```python
from build123d import *

# Parameters (mm, degrees)
BOSS_EXTRUDE1_DEPTH = 2.5
BOSS_EXTRUDE3_START = 2.5
BOSS_EXTRUDE3_DEPTH = 3
BOSS_EXTRUDE2_DEPTH = 7


with BuildPart() as part:
    # Sketch1 → Boss-Extrude1 (new body)
    with BuildSketch(Plane.XY):
        with BuildLine():
            ThreePointArc((-43.2, -11.688179282), (-41.735533906, -15.223713187), (-38.2, -16.688179282))
            Line((-38.2, -16.688179282), (-5, -16.688179282))
            Line((-5, -16.688179282), (-5, 5.203986913))
            Line((-5, 5.203986913), (-35.346679904, 16.688179282))
            Line((-35.346679904, 16.688179282), (-38.2, 16.688179282))
            ThreePointArc((-38.2, 16.688179282), (-41.735533906, 15.223713187), (-43.2, 11.688179282))
            Line((-43.2, 11.688179282), (-43.2, -11.688179282))
        make_face()
        with BuildLine():
            ThreePointArc((-41.2, 11.338179282), (-37.85, 14.688179282), (-34.5, 11.338179282))
            Line((-34.5, 11.338179282), (-34.5, 1.338179282))
            ThreePointArc((-34.5, 1.338179282), (-37.85, -2.011820718), (-41.2, 1.338179282))
            Line((-41.2, 1.338179282), (-41.2, 11.338179282))
        make_face(mode=Mode.SUBTRACT)
        with BuildLine():
            Line((-41.2, 11.338179282), (-41.2, 1.338179282))
            ThreePointArc((-41.2, 1.338179282), (-37.85, -2.011820718), (-34.5, 1.338179282))
            Line((-34.5, 1.338179282), (-34.5, 11.338179282))
            ThreePointArc((-34.5, 11.338179282), (-37.85, 14.688179282), (-41.2, 11.338179282))
        make_face()
        with BuildLine():
            Line((5, 5.203986913), (5, -16.688179282))
            Line((5, -16.688179282), (38.2, -16.688179282))
            ThreePointArc((38.2, -16.688179282), (41.735533906, -15.223713187), (43.2, -11.688179282))
            Line((43.2, -11.688179282), (43.2, 11.688179282))
            ThreePointArc((43.2, 11.688179282), (41.735533906, 15.223713187), (38.2, 16.688179282))
            Line((38.2, 16.688179282), (35.346679904, 16.688179282))
            Line((35.346679904, 16.688179282), (5, 5.203986913))
        make_face()
        with BuildLine():
            ThreePointArc((34.5, 11.338179282), (37.85, 14.688179282), (41.2, 11.338179282))
            Line((41.2, 11.338179282), (41.2, 1.338179282))
            ThreePointArc((41.2, 1.338179282), (37.85, -2.011820718), (34.5, 1.338179282))
            Line((34.5, 1.338179282), (34.5, 11.338179282))
        make_face(mode=Mode.SUBTRACT)
        with BuildLine():
            Line((34.5, 11.338179282), (34.5, 1.338179282))
            ThreePointArc((34.5, 1.338179282), (37.85, -2.011820718), (41.2, 1.338179282))
            Line((41.2, 1.338179282), (41.2, 11.338179282))
            ThreePointArc((41.2, 11.338179282), (37.85, 14.688179282), (34.5, 11.338179282))
        make_face()
    extrude(amount=BOSS_EXTRUDE1_DEPTH)

    # Sketch1<4> → Boss-Extrude3 (add)
    with BuildSketch(Plane.XY.offset(BOSS_EXTRUDE3_START)):
        with BuildLine():
            ThreePointArc((-43.2, -11.688179282), (-41.735533906, -15.223713187), (-38.2, -16.688179282))
            Line((-38.2, -16.688179282), (-5, -16.688179282))
            Line((-5, -16.688179282), (-5, 5.203986913))
            Line((-5, 5.203986913), (-35.346679904, 16.688179282))
            Line((-35.346679904, 16.688179282), (-38.2, 16.688179282))
            ThreePointArc((-38.2, 16.688179282), (-41.735533906, 15.223713187), (-43.2, 11.688179282))
            Line((-43.2, 11.688179282), (-43.2, -11.688179282))
        make_face()
        with BuildLine():
            ThreePointArc((-41.2, 11.338179282), (-37.85, 14.688179282), (-34.5, 11.338179282))
            Line((-34.5, 11.338179282), (-34.5, 1.338179282))
            ThreePointArc((-34.5, 1.338179282), (-37.85, -2.011820718), (-41.2, 1.338179282))
            Line((-41.2, 1.338179282), (-41.2, 11.338179282))
        make_face(mode=Mode.SUBTRACT)
        Polygon((-5, 5.203986913), (-5, -16.688179282), (5, -16.688179282), (5, 5.203986913), (0, 3.311820718), align=None)
        with BuildLine():
            Line((5, 5.203986913), (5, -16.688179282))
            Line((5, -16.688179282), (38.2, -16.688179282))
            ThreePointArc((38.2, -16.688179282), (41.735533906, -15.223713187), (43.2, -11.688179282))
            Line((43.2, -11.688179282), (43.2, 11.688179282))
            ThreePointArc((43.2, 11.688179282), (41.735533906, 15.223713187), (38.2, 16.688179282))
            Line((38.2, 16.688179282), (35.346679904, 16.688179282))
            Line((35.346679904, 16.688179282), (5, 5.203986913))
        make_face()
        with BuildLine():
            ThreePointArc((34.5, 11.338179282), (37.85, 14.688179282), (41.2, 11.338179282))
            Line((41.2, 11.338179282), (41.2, 1.338179282))
            ThreePointArc((41.2, 1.338179282), (37.85, -2.011820718), (34.5, 1.338179282))
            Line((34.5, 1.338179282), (34.5, 11.338179282))
        make_face(mode=Mode.SUBTRACT)
        with BuildLine():
            Line((34.5, 11.338179282), (34.5, 1.338179282))
            ThreePointArc((34.5, 1.338179282), (37.85, -2.011820718), (41.2, 1.338179282))
            Line((41.2, 1.338179282), (41.2, 11.338179282))
            ThreePointArc((41.2, 11.338179282), (37.85, 14.688179282), (34.5, 11.338179282))
        make_face()
        with BuildLine():
            Line((-41.2, 11.338179282), (-41.2, 1.338179282))
            ThreePointArc((-41.2, 1.338179282), (-37.85, -2.011820718), (-34.5, 1.338179282))
            Line((-34.5, 1.338179282), (-34.5, 11.338179282))
            ThreePointArc((-34.5, 11.338179282), (-37.85, 14.688179282), (-41.2, 11.338179282))
        make_face()
    extrude(amount=BOSS_EXTRUDE3_DEPTH)

    # Sketch1<3> → Boss-Extrude2 (add)
    with BuildSketch(Plane.XY):
        with BuildLine():
            Line((34.5, 11.338179282), (34.5, 1.338179282))
            ThreePointArc((34.5, 1.338179282), (37.85, -2.011820718), (41.2, 1.338179282))
            Line((41.2, 1.338179282), (41.2, 11.338179282))
            ThreePointArc((41.2, 11.338179282), (37.85, 14.688179282), (34.5, 11.338179282))
        make_face()
        with BuildLine():
            Line((-41.2, 11.338179282), (-41.2, 1.338179282))
            ThreePointArc((-41.2, 1.338179282), (-37.85, -2.011820718), (-34.5, 1.338179282))
            Line((-34.5, 1.338179282), (-34.5, 11.338179282))
            ThreePointArc((-34.5, 11.338179282), (-37.85, 14.688179282), (-41.2, 11.338179282))
        make_face()
    extrude(amount=-BOSS_EXTRUDE2_DEPTH)


solid = part.part
```
Geometry check sheet. Reference: the model listing, model coordinates, mm. A direction names the side the tool comes from. Give positions to 0.01 mm unless a question says otherwise; leave off trailing zeros. Write each loop counter-clockwise with the first axis right and the second up, starting at its lowest first coordinate (ties: lowest second). Pieces come first, ordered by that corner, then holes.
1) Material ranges on L1, parallel to X at y = -2.5, z = 1.25; L2, parallel to Z at x = 13, y = -4; L3, parallel to X at y = -1.5, z = -1.75, recorded low to high.
2) Release check for a two-part mould opening along X. For faces 1 (the flat face through (5, -6, 1)), 2 (the cylindrical face through (37.78, -2.01, -3.45)), 3 (the cylindrical face through (-41.774, -15.185, 2.712)), 4 (the flat face through (-37, 16.688, 3)) record: pulls with the +X half, pulls with the -X half, needs draft (parallel to the pull), parting line crosses it, or undercut.
3) Section check B-B, the plane y = 2.5. Record the boundary of the cut face in (x, z), and give its area (3 significant figures).
4) Section check A-A, the plane z = -5. Record the boundary of the cut face in (x, y), and give its area (3 significant figures).
5) Access from +Z, -Z, +X, -X, +Y, -Y to the whole of each face (thin tool, end or side, straight path). Record for faces 5 (the flat face through (41.2, 6, -3)), 6 (the flat face through (0, -6, 2.5)), 7 (the cylindrical face through (-37.92, -2.01, -3.45)).
6) Section check C-C, the plane y = 13. Record the boundary of the cut face in (x, z).
7) Section check D-D, the plane x = -3.5. Record the boundary of the cut face in (y, z), and give its area (3 significant figures).
8) Gauge pin test, flat ends, axial feed: pin 1 (8 mm diameter, centred on x = -0.5, y = -6.5, fed in from -Z); pin 2 (2 mm diameter, centred on y = 5, z = -3, fed in from +X); pin 3 (3.5 mm diameter, centred on y = 6.5, z = -4, fed in from -X). Record the tip position at first contact, or that the pin passes through.
Computed:
1. L1: x = -43.2 to -5, 5 to 43.2
1. L2: z = 0 to 5.5
1. L3: x = -39.63 to -36.07, 36.07 to 39.63
2. face 1: undercut
2. face 2: undercut
2. face 3: pulls with the -X half
2. face 4: needs draft
3. outline: (-43.2, 0) - (-41.2, 0) - (-41.2, -7) - (-34.5, -7) - (-34.5, 0) - (-5, 0) - (-5, 2.5) - (5, 2.5) - (5, 0) - (34.5, 0) - (34.5, -7) - (41.2, -7) - (41.2, 0) - (43.2, 0) - (43.2, 5.5) - (-43.2, 5.5) - close
3. area: 544 mm2
4. outline: (-41.2, 1.34) arc R3.35 ccw to (-34.5, 1.34) - (-34.5, 11.34) arc R3.35 ccw to (-41.2, 11.34) - close; (34.5, 1.34) arc R3.35 ccw to (41.2, 1.34) - (41.2, 11.34) arc R3.35 ccw to (34.5, 11.34) - close
4. area: 205 mm2
5. face 5: -Z, +X, +Y, -Y
5. face 6: -Z, +Y, -Y
5. face 7: -Z, -Y
6. outline: (-43.02, 0) - (-40.76, 0) - (-40.76, -7) - (-34.94, -7) - (-34.94, 0) - (-25.6, 0) - (-25.6, 5.5) - (-43.02, 5.5) - close; (25.6, 0) - (34.94, 0) - (34.94, -7) - (40.76, -7) - (40.76, 0) - (43.02, 0) - (43.02, 5.5) - (25.6, 5.5) - close
7. outline: (-16.69, 2.5) - (4.64, 2.5) - (4.64, 5.5) - (-16.69, 5.5) - close
7. area: 64.0 mm2
8. pin 1: stops at z = 2.5
8. pin 2: stops at x = 41.2
8. pin 3: stops at x = -41.2
